from build123d import *

# Parameters (mm, degrees)
SKETCH1_W           = 60
SKETCH1_H           = 60
SKETCH1_R           = 2.75
SKETCH1_R_2         = 4.15
BOSS_EXTRUDE1_DEPTH = 2
CHAMFER1_SIZE       = 1
CHAMFER2_SIZE       = 1
FILLET1_R           = 5


with BuildPart() as part:
    # Sketch1 → Boss-Extrude1 (new body)
    with BuildSketch(Plane(origin=(0, 0, 0), x_dir=(1, 0, 0), z_dir=(0, 1, 0))):
        Rectangle(SKETCH1_W, SKETCH1_H)
        with Locations(Location((23.57, -23.57, 0), (0, 0, 270))):
            Circle(SKETCH1_R, mode=Mode.SUBTRACT)
        with Locations(Location((-23.57, -23.57, 0), (0, 0, 270))):
            Circle(SKETCH1_R, mode=Mode.SUBTRACT)
        with Locations(Location((-23.57, 23.57, 0), (0, 0, 270))):
            Circle(SKETCH1_R, mode=Mode.SUBTRACT)
        with Locations(Location((23.57, 23.57, 0), (0, 0, 270))):
            Circle(SKETCH1_R, mode=Mode.SUBTRACT)
        with Locations(Location((0, 0, 0), (0, 0, 270))):
            Circle(SKETCH1_R_2, mode=Mode.SUBTRACT)
    extrude(amount=BOSS_EXTRUDE1_DEPTH)

    # Chamfer1
    chamfer1_edges = [part.edges().sort_by_distance(p)[0] for p in [
        (23.57, 2, 20.82),
        (-23.57, 2, 20.82),
        (-23.57, 2, -26.32),
        (23.57, 2, -26.32),
    ]]
    chamfer(chamfer1_edges, length=CHAMFER1_SIZE)

    # Chamfer2
    chamfer2_edges = [part.edges().sort_by_distance(p)[0] for p in [
        (0, 0, -4.15),
    ]]
    chamfer(chamfer2_edges, length=CHAMFER2_SIZE)

    # Fillet1
    fillet1_edges = [part.edges().sort_by_distance(p)[0] for p in [
        (30, 1, 30),
        (-30, 1, 30),
        (-30, 1, -30),
        (30, 1, -30),
    ]]
    fillet(fillet1_edges, radius=FILLET1_R)


solid = part.part
The listing builds one solid part. Answer for the finished solid, in the listing's coordinates (mm). Round coordinates to 2 decimals unless told otherwise and drop trailing zeros. Loops run counter-clockwise (first coordinate to the right, second up) from the corner with the lowest first, then second, coordinate; pieces in that order, holes last. Notation, with made-up numbers: M -40,11 L -15,11 A22 ccw -15,39 Z; hole C -13.75,-20.5 d6. An arc over 180 degrees is marked long. Write each question's results on one line, items separated by ' | '. Start each with the question number.
1) Find section A-A on z = 0. Write down the section's boundary in (x, y), plus the area to 3 significant figures.
2) Find section B-B on z = -23.57. Write down the section's boundary in (x, y), plus the area to 3 significant figures.
3) Straight lines are drawn through the part: probe 1 along X at (y, z) = (0.6, 23.57); probe 2 along X at (y, z) = (1.55, 0); probe 3 along X at (y, z) = (0.2, -22). For each, find the intervals that lie inside material, in ascending order.
4) Determine the mould class of faces 1 (the flat face through (-30, 1, 0)), 2 (the cylindrical face through (28, 1, -29)), 3 (the flat face through (0, 1, -30)), 4 (the cylindrical face through (21.13, 0.49, 24.84)) for opening direction X: pulls with the +X half, pulls with the -X half, needs draft (parallel to the pull), parting line crosses it, or undercut.
5) Find section C-C on x = 23.57. Write down the section's boundary in (y, z).
Final values:
1) outline: M -30,0 L -5.15,0 L -4.15,1 L -4.15,2 L -30,2 Z; M 4.15,1 L 5.15,0 L 30,0 L 30,2 L 4.15,2 Z | area: 102 mm²
2) outline: M -30,0 L -26.32,0 L -26.32,1 L -27.32,2 L -30,2 Z; M -20.82,0 L 20.82,0 L 20.82,1 L 19.82,2 L -19.82,2 L -20.82,1 Z; M 26.32,0 L 30,0 L 30,2 L 27.32,2 L 26.32,1 Z | area: 96.0 mm²
3) probe 1: -30 to -26.32, -20.82 to 20.82, 26.32 to 30 | probe 2: -30 to -4.15, 4.15 to 30 | probe 3: -30 to -25.83, -21.31 to 21.31, 25.83 to 30
4) face 1: pulls with the -X half | face 2: pulls with the +X half | face 3: needs draft | face 4: undercut
5) outline: M 0,-30 L 2,-30 L 2,-27.32 L 1,-26.32 L 0,-26.32 Z; M 0,-20.82 L 1,-20.82 L 2,-19.82 L 2,19.82 L 1,20.82 L 0,20.82 Z; M 0,26.32 L 1,26.32 L 2,27.32 L 2,30 L 0,30 Z
